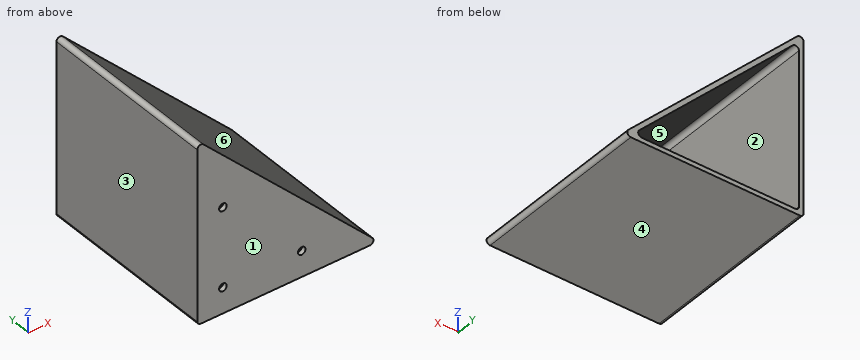
from build123d import *

# Parameters (mm, degrees)
BOSS_EXTRUDE1_DEPTH         = 100
SHELL1_T                    = -2.5
TAP_DRILL_FOR_M5X0_8_TAP1_D = 4.2
FILLET1_R                   = 2


with BuildPart() as part:
    # Sketch1 → Boss-Extrude1 (new body)
    with BuildSketch(Plane(origin=(0, 0, 0), x_dir=(1, 0, 0), z_dir=(0, 1, 0))):
        Polygon((0, 0), (0, -100), (100, 0), align=None)
    extrude(amount=BOSS_EXTRUDE1_DEPTH)

    # Shell1
    shell1_openings = [part.faces().sort_by_distance(p)[0] for p in [
        (33.333333333, 100, 33.333333333),
    ]]
    offset(amount=SHELL1_T, openings=shell1_openings, kind=Kind.INTERSECTION)

    # Tap Drill for M5x0.8 Tap1 (through all)
    with Locations(Plane(origin=(14.142135624, 2.5, 14.142135624), x_dir=(0, 0, 1), z_dir=(0, 1, 0))):
        with Locations((0, 0), (43.431457505, 0), (0, 43.431457505)):
            Hole(TAP_DRILL_FOR_M5X0_8_TAP1_D / 2)

    # Fillet1
    fillet1_edges = [part.edges().sort_by_distance(p)[0] for p in [
        (93.964466094, 51.25, 2.5),
        (2.5, 51.25, 2.5),
        (2.5, 51.25, 93.964466094),
        (100, 50, 0),
        (0, 50, 100),
        (0, 50, 0),
    ]]
    fillet(fillet1_edges, radius=FILLET1_R)


solid = part.part
Geometry check sheet. Reference: the model listing, model coordinates, mm. Face numbers are marked on the shaded views. A direction names the side the tool comes from. Coordinates: 2 decimals unless noted, no trailing zeros. Loops run counter-clockwise (first coordinate to the right, second up) from the corner with the lowest first, then second, coordinate; pieces in that order, holes last. Notation, with made-up numbers: (-28, 39.25) - (-2, 39.25) arc R14 ccw to (-2, 46.25) - close; hole circle Ø6 at (37, -13). An arc over 180 degrees is marked (long way). Use one line per item in the form item = value. Start each with the question number.
Item 1: Section check C-C, the plane x = 51. Enter the section's corners in (y, z), and give its area (3 significant figures).
Item 2: Gauge pin test, flat ends, axial feed: pin 1 (1 mm diameter, centred on x = 69.5, y = 16, fed in from +Z); pin 2 (1 mm diameter, centred on y = 79.5, z = 50, fed in from +X); pin 3 (8 mm diameter, centred on x = 38, y = 12.5, fed in from +Z). Record the tip position at first contact, or that the pin passes through.
Item 3: Mould release check, pull along Z, two halves, no side actions. Record for the marked faces 3, 4, 5 and 6: +Z half, -Z half, draft (parallel to the pull), parting line (faces both ways), or undercut.
Item 4: Section check D-D, the plane z = 57. Enter the section's corners in (x, y).
Item 5: Thickness scan on probe 1 along X at (y, z) = (36.5, 82); probe 2 along X at (y, z) = (75.5, 90); probe 3 along Z at (x, y) = (13, 19.5). Record the ranges inside material, lowest first.
Item 6: Section check A-A, the plane y = 71.5. Enter the section's corners in (x, z).
Item 7: Section check B-B, the plane z = 36.5. Enter the section's corners in (x, y).
Item 8: Tool access check on the marked faces 1 and 2. Record the directions out of +Z, -Z, +X, -X, +Y, -Y that give a thin tool (end or side, any length) a straight path to the whole face; none if there is none.
Computed:
q1.outline = (0, 0) - (100, 0) - (100, 2.5) - (2.5, 2.5) - (2.5, 45.46) - (100, 45.46) - (100, 49) - (0, 49) - close
q1.area = 711 mm2
q2.pin_1 = 31
q2.pin_2 = 50.5
q2.pin_3 = 66
q3.face_3 = draft
q3.face_4 = -Z half
q3.face_5 = undercut
q3.face_6 = +Z half
q4.outline = (0, 0) - (12.12, 0) - (12.12, 2.5) - (2.5, 2.5) - (2.5, 100) - (0, 100) - close; (16.16, 0) - (43, 0) - (43, 100) - (39.46, 100) - (39.46, 2.5) - (16.16, 2.5) - close
q5.probe_1 = 0 to 2.5, 14.46 to 18
q5.probe_2 = 0 to 2.7, 6.46 to 10
q5.probe_3 = 0 to 2.5, 83.46 to 87
q6.outline = (0, 2) arc R2 ccw to (2, 0) - (95.17, 0) arc R2 ccw to (96.59, 3.41) - (3.41, 96.59) arc R2 ccw to (0, 95.17) - close; hole (2.5, 4.5) arc R2 ccw to (4.5, 2.5) - (89.14, 2.5) arc R2 ccw to (90.55, 5.91) - (5.91, 90.55) arc R2 ccw to (2.5, 89.14) - close
q7.outline = (0, 0) - (63.5, 0) - (63.5, 100) - (59.96, 100) - (59.96, 2.5) - (2.5, 2.5) - (2.5, 100) - (0, 100) - close
q8.face_1 = +Z, -Z, +X, -X, -Y
q8.face_2 = +Y
